```python
from build123d import *

# Parameters (mm, degrees)
ESQUISSE1_W        = 32
ESQUISSE1_H        = 32
BOSS_EXTRU_1_DEPTH = 1.25
ESQUISSE2_W        = 7.5
ESQUISSE2_H        = 3.7
BOSS_EXTRU_2_DEPTH = 5
BOSS_EXTRU_3_DEPTH = 3.5
ESQUISSE4_R        = 6.5
BOSS_EXTRU_4_DEPTH = 14
ESQUISSE5_R        = 9
BOSS_EXTRU_5_DEPTH = 5


with BuildPart() as part:
    # Esquisse1 → Boss.-Extru.1 (new body)
    with BuildSketch(Plane.XY):
        Rectangle(ESQUISSE1_W, ESQUISSE1_H)
        with BuildLine():
            Line((-13.171572875, 15.116116524), (-12.464466094, 14.409009742))
            ThreePointArc((-12.464466094, 14.409009742), (-12.464466094, 12.464466094), (-14.409009742, 12.464466094))
            Line((-14.409009742, 12.464466094), (-15.116116524, 13.171572875))
            ThreePointArc((-15.116116524, 13.171572875), (-15.116116524, 15.116116524), (-13.171572875, 15.116116524))
        make_face(mode=Mode.SUBTRACT)
        with BuildLine():
            Line((15.116116524, 13.171572875), (14.409009742, 12.464466094))
            ThreePointArc((14.409009742, 12.464466094), (12.464466094, 12.464466094), (12.464466094, 14.409009742))
            Line((12.464466094, 14.409009742), (13.171572875, 15.116116524))
            ThreePointArc((13.171572875, 15.116116524), (15.116116524, 15.116116524), (15.116116524, 13.171572875))
        make_face(mode=Mode.SUBTRACT)
        with BuildLine():
            Line((13.171572875, -15.116116524), (12.464466094, -14.409009742))
            ThreePointArc((12.464466094, -14.409009742), (12.464466094, -12.464466094), (14.409009742, -12.464466094))
            Line((14.409009742, -12.464466094), (15.116116524, -13.171572875))
            ThreePointArc((15.116116524, -13.171572875), (15.116116524, -15.116116524), (13.171572875, -15.116116524))
        make_face(mode=Mode.SUBTRACT)
        with BuildLine():
            Line((-15.116116524, -13.171572875), (-14.409009742, -12.464466094))
            ThreePointArc((-14.409009742, -12.464466094), (-12.464466094, -12.464466094), (-12.464466094, -14.409009742))
            Line((-12.464466094, -14.409009742), (-13.171572875, -15.116116524))
            ThreePointArc((-13.171572875, -15.116116524), (-15.116116524, -15.116116524), (-15.116116524, -13.171572875))
        make_face(mode=Mode.SUBTRACT)
    extrude(amount=BOSS_EXTRU_1_DEPTH)

    # Esquisse2 → Boss.-Extru.2 (add)
    with BuildSketch(Plane.XY.offset(1.25)):
        with Locations((6.9, -14.15)):
            Rectangle(ESQUISSE2_W, ESQUISSE2_H)
    extrude(amount=BOSS_EXTRU_2_DEPTH)

    # Esquisse3 → Boss.-Extru.3 (add)
    with BuildSketch(Plane(origin=(0, 0, 0), x_dir=(-1, 0, 0), z_dir=(0, 0, -1))):
        with BuildLine():
            Line((-6.5, 6.5), (6.5, 6.5))
            Line((6.5, 6.5), (6.5, 2))
            Line((6.5, 2), (8.5, 2))
            ThreePointArc((8.5, 2), (10.5, 0), (8.5, -2))
            Line((8.5, -2), (6.5, -2))
            Line((6.5, -2), (6.5, -6.5))
            Line((6.5, -6.5), (-6.5, -6.5))
            Line((-6.5, -6.5), (-6.5, -2))
            Line((-6.5, -2), (-8.5, -2))
            ThreePointArc((-8.5, -2), (-10.5, 0), (-8.5, 2))
            Line((-8.5, 2), (-6.5, 2))
            Line((-6.5, 2), (-6.5, 6.5))
        make_face()
    extrude(amount=BOSS_EXTRU_3_DEPTH)

    # Esquisse4 → Boss.-Extru.4 (add)
    with BuildSketch(Plane(origin=(0, 0, -3.5), x_dir=(-1, 0, 0), z_dir=(0, 0, -1))):
        with Locations(Location((0, 0, 0), (0, 0, 270))):
            Circle(ESQUISSE4_R)
    extrude(amount=BOSS_EXTRU_4_DEPTH)

    # Esquisse5 → Boss.-Extru.5 (add)
    with BuildSketch(Plane(origin=(0, 0, -17.5), x_dir=(-1, 0, 0), z_dir=(0, 0, -1))):
        Circle(ESQUISSE5_R)
    extrude(amount=BOSS_EXTRU_5_DEPTH)

    # Esquisse6 → Révolution2 (revolve)
    with BuildSketch(Plane(origin=(0, 0, 0), x_dir=(0, 0, -1), z_dir=(1, 0, 0))):
        with BuildLine():
            Line((22.5, 0), (24.5, 0))
            ThreePointArc((24.5, 0), (23.993975029, 4.609772229), (22.5, 9))
            Line((22.5, 9), (22.5, 0))
        make_face()
    revolve(axis=Axis((0, 0, -22.5), (0, 0, -1)))


solid = part.part
```
Model file for the job. Use its own axes, mm. A direction names the side the tool comes from. Round coordinates to 2 decimals unless told otherwise and drop trailing zeros. Write each loop counter-clockwise with the first axis right and the second up, starting at its lowest first coordinate (ties: lowest second). Pieces come first, ordered by that corner, then holes. Notation, with made-up numbers: M -30.5,-6 L 22.5,-6 A13 ccw 22.5,-2 Z; hole C 70,-28.5 d10. An arc over 180 degrees is marked long. Put each result on its own line as item: value.
Item 1: Cut at B-B (y = 0). List the corners of the cut face in (x, z), and give its area (3 significant figures).
Responses:
outline: M -16,0 L -10.5,0 L -10.5,-3.5 L -6.5,-3.5 L -6.5,-17.5 L -9,-17.5 L -9,-22.5 A21.25 ccw 9,-22.5 L 9,-17.5 L 6.5,-17.5 L 6.5,-3.5 L 10.5,-3.5 L 10.5,0 L 16,0 L 16,1.25 L -16,1.25 Z
area: 410 mm²
Item 2: Flat gauge pins, fed straight in: P1, Ø4, axis at y = -3.5, z = -2.5, coming from the +X side; P2, Ø1, axis at y = -4, z = -21.5, coming from the -X side; P3, Ø1.8, axis at x = 1.5, z = -2.5, coming from the +Y side. Where does each tip first touch, or does it go through?
Responses:
P1: x = 9.82
P2: x = -8.29
P3: y = 6.5
Item 3: Cut at A-A (x = 7). List the corners of the cut face in (y, z).
Responses:
outline: M -16,0 L -2,0 L -2,-3.5 L 2,-3.5 L 2,0 L 16,0 L 16,1.25 L -12.3,1.25 L -12.3,6.25 L -16,6.25 Z; M -5.66,-22.5 A20.06 ccw 5.66,-22.5 L 5.66,-17.5 L -5.66,-17.5 Z
Item 4: Mould opens along X. For faces 4 (the cylindrical face through (-12.44, 12.49, 0.62)), 5 (the flat face through (3.15, -14, 4)), 6 (the cylindrical face through (1.172, 8.923, -19.965)), 7 (the flat face through (-7, 0, -3.5)) say: +X half, -X half, draft (parallel to the pull), parting line (faces both ways), or undercut.
Responses:
face 4: undercut
face 5: -X half
face 6: parting line
face 7: draft
Item 5: Tool access for faces 1 (the flat face through (0, 6.5, -2)), 2 (the cylindrical face through (3.955, 5.158, -10.402)), 3 (the flat face through (-6.5, -4, -2)): list every direction of +Z, -Z, +X, -X, +Y, -Y with a clear straight run to the whole face (end or side of a thin tool).
Responses:
face 1: +X, -X, +Y
face 2: none
face 3: -X, -Y
Item 6: Cut at D-D (x = -3). List the corners of the cut face in (y, z), and give its area (3 significant figures).
Responses:
outline: M -16,0 L -6.5,0 L -6.5,-3.5 L -5.77,-3.5 L -5.77,-17.5 L -8.49,-17.5 L -8.49,-22.5 A21.04 ccw 8.49,-22.5 L 8.49,-17.5 L 5.77,-17.5 L 5.77,-3.5 L 6.5,-3.5 L 6.5,0 L 16,0 L 16,1.25 L -16,1.25 Z
area: 352 mm²
Item 7: Cut at C-C (z = -2.5). List the corners of the cut face in (x, y), and give its area (3 significant figures).
Responses:
outline: M -8.5,-2 L -6.5,-2 L -6.5,-6.5 L 6.5,-6.5 L 6.5,-2 L 8.5,-2 A2 ccw 8.5,2 L 6.5,2 L 6.5,6.5 L -6.5,6.5 L -6.5,2 L -8.5,2 A2 ccw Z
area: 198 mm²
Item 8: Probe L1, parallel to X at y = -2.5, z = -0.5; L2, parallel to Z at x = 9.5, y = 3; L3, parallel to Z at x = -7, y = -4. List the from-to ranges inside material, lowest first. Write a range as from..to.
Responses:
L1: -6.5..6.5
L2: 0..1.25
L3: -22.91..-17.5, 0..1.25
